Work out the finished part from the listing and answer in its coordinate system (mm). Face numbers are marked on the shaded views. A direction names the side the tool comes from. Give positions to 0.01 mm unless a question says otherwise; leave off trailing zeros. Order: outer loops, then holes, each group sorted by start corner. A loop starts at its lowest first (then second) coordinate and runs counter-clockwise, first axis right, second up. Notation, with made-up numbers: M -26.75,36 L 5.25,36 A18 ccw 5.25,49 Z; hole C 22.5,85 d5. An arc over 180 degrees is marked long. One line per item, written item: value.
from build123d import *

# Parameters (mm, degrees)
F0_W     = 86.995
F0_H     = 86.995
F1_DEPTH = 1.5875
F2_W     = 86.995
F2_H     = 86.995
F2_W_2   = 83.82
F2_H_2   = 83.82
F3_DEPTH = 31.75
F4_R     = 1.7145
F5_DEPTH = 17.78
F6_R     = 2.54
F7_DEPTH = 1.5875


with BuildPart() as f1:
    # F0 (on Top) → F1 (new body)
    with BuildSketch(Plane.XY):
        Rectangle(F0_W, F0_H)
    extrude(amount=F1_DEPTH)

    # F2 (on face) → F3 (join)
    with BuildSketch(Plane.XY.offset(1.5875)):
        Rectangle(F2_W, F2_H)
        Rectangle(F2_W_2, F2_H_2, mode=Mode.SUBTRACT)
    extrude(amount=F3_DEPTH)

    # F4 (on face) → F5 (join)
    with BuildSketch(Plane.XY.offset(1.5875)):
        with BuildLine():
            ThreePointArc((-24.60625, -30.4176050998), (-21.5374457933, -28.6995567884), (-20.32, -25.4))
            ThreePointArc((-20.32, -25.4), (-25.0019007077, -20.3356227477), (-30.4176050998, -24.60625))
            Line((-30.4176050998, -24.60625), (-30.4176050998, -26.19375))
            ThreePointArc((-30.4176050998, -26.19375), (-28.9921024484, -28.9921024484), (-26.19375, -30.4176050998))
            Line((-26.19375, -30.4176050998), (-24.60625, -30.4176050998))
        make_face()
        with Locations((-25.4, -25.4)):
            Circle(F4_R, mode=Mode.SUBTRACT)
        with BuildLine():
            Line((-30.4176050998, -26.19375), (-30.4176050998, -24.60625))
            ThreePointArc((-30.4176050998, -24.60625), (-30.48, -25.4), (-30.4176050998, -26.19375))
        make_face()
        with BuildLine():
            ThreePointArc((-30.4176050998, -26.19375), (-30.48, -25.4), (-30.4176050998, -24.60625))
            Line((-30.4176050998, -24.60625), (-41.91, -24.60625))
            Line((-41.91, -24.60625), (-41.91, -26.19375))
            Line((-41.91, -26.19375), (-30.4176050998, -26.19375))
        make_face()
        with BuildLine():
            Line((-24.60625, -41.91), (-24.60625, -30.4176050998))
            ThreePointArc((-24.60625, -30.4176050998), (-25.4, -30.48), (-26.19375, -30.4176050998))
            Line((-26.19375, -30.4176050998), (-26.19375, -41.91))
            Line((-26.19375, -41.91), (-24.60625, -41.91))
        make_face()
        with BuildLine():
            ThreePointArc((-26.19375, -30.4176050998), (-25.4, -30.48), (-24.60625, -30.4176050998))
            Line((-24.60625, -30.4176050998), (-26.19375, -30.4176050998))
        make_face()
        with BuildLine():
            ThreePointArc((-30.4176050998, 24.60625), (-25.0019007077, 20.3356227477), (-20.32, 25.4))
            ThreePointArc((-20.32, 25.4), (-21.5374457933, 28.6995567884), (-24.60625, 30.4176050998))
            ThreePointArc((-24.60625, 30.4176050998), (-25.4, 30.48), (-26.19375, 30.4176050998))
            ThreePointArc((-26.19375, 30.4176050998), (-28.9921024484, 28.9921024484), (-30.4176050998, 26.19375))
            ThreePointArc((-30.4176050998, 26.19375), (-30.48, 25.4), (-30.4176050998, 24.60625))
        make_face()
        with Locations((-25.4, 25.4)):
            Circle(F4_R, mode=Mode.SUBTRACT)
        with BuildLine():
            ThreePointArc((-26.19375, 30.4176050998), (-25.4, 30.48), (-24.60625, 30.4176050998))
            Line((-24.60625, 30.4176050998), (-24.60625, 41.91))
            Line((-24.60625, 41.91), (-26.19375, 41.91))
            Line((-26.19375, 41.91), (-26.19375, 30.4176050998))
        make_face()
        with BuildLine():
            Line((-41.91, 24.60625), (-30.4176050998, 24.60625))
            ThreePointArc((-30.4176050998, 24.60625), (-30.48, 25.4), (-30.4176050998, 26.19375))
            Line((-30.4176050998, 26.19375), (-41.91, 26.19375))
            Line((-41.91, 26.19375), (-41.91, 24.60625))
        make_face()
        with BuildLine():
            Line((24.60625, -41.91), (26.19375, -41.91))
            Line((26.19375, -41.91), (26.19375, -30.4176050998))
            ThreePointArc((26.19375, -30.4176050998), (25.4, -30.48), (24.60625, -30.4176050998))
            Line((24.60625, -30.4176050998), (24.60625, -41.91))
        make_face()
        with BuildLine():
            ThreePointArc((24.60625, -30.4176050998), (25.4, -30.48), (26.19375, -30.4176050998))
            ThreePointArc((26.19375, -30.4176050998), (28.9921024484, -28.9921024484), (30.4176050998, -26.19375))
            ThreePointArc((30.4176050998, -26.19375), (30.4643772523, -25.7980992923), (30.48, -25.4))
            ThreePointArc((30.48, -25.4), (30.4643772523, -25.0019007077), (30.4176050998, -24.60625))
            ThreePointArc((30.4176050998, -24.60625), (21.8078975516, -21.8078975516), (24.60625, -30.4176050998))
        make_face()
        with Locations((25.4, -25.4)):
            Circle(F4_R, mode=Mode.SUBTRACT)
        with BuildLine():
            ThreePointArc((30.48, -25.4), (30.4643772523, -25.7980992923), (30.4176050998, -26.19375))
            Line((30.4176050998, -26.19375), (41.91, -26.19375))
            Line((41.91, -26.19375), (41.91, -24.60625))
            Line((41.91, -24.60625), (30.4176050998, -24.60625))
            ThreePointArc((30.4176050998, -24.60625), (30.4643772523, -25.0019007077), (30.48, -25.4))
        make_face()
        with BuildLine():
            Line((30.4176050998, 24.60625), (41.91, 24.60625))
            Line((41.91, 24.60625), (41.91, 26.19375))
            Line((41.91, 26.19375), (30.4176050998, 26.19375))
            ThreePointArc((30.4176050998, 26.19375), (30.4643772523, 25.7980992923), (30.48, 25.4))
            ThreePointArc((30.48, 25.4), (30.4643772523, 25.0019007077), (30.4176050998, 24.60625))
        make_face()
        with BuildLine():
            ThreePointArc((24.60625, 30.4176050998), (21.8078975516, 21.8078975516), (30.4176050998, 24.60625))
            ThreePointArc((30.4176050998, 24.60625), (30.4643772523, 25.0019007077), (30.48, 25.4))
            ThreePointArc((30.48, 25.4), (30.4643772523, 25.7980992923), (30.4176050998, 26.19375))
            ThreePointArc((30.4176050998, 26.19375), (28.9921024484, 28.9921024484), (26.19375, 30.4176050998))
            ThreePointArc((26.19375, 30.4176050998), (25.4, 30.48), (24.60625, 30.4176050998))
        make_face()
        with Locations((25.4, 25.4)):
            Circle(F4_R, mode=Mode.SUBTRACT)
        with BuildLine():
            Line((24.60625, 41.91), (24.60625, 30.4176050998))
            ThreePointArc((24.60625, 30.4176050998), (25.4, 30.48), (26.19375, 30.4176050998))
            Line((26.19375, 30.4176050998), (26.19375, 41.91))
            Line((26.19375, 41.91), (24.60625, 41.91))
        make_face()
    extrude(amount=F5_DEPTH)

    # F6 (on face) → F7 (cut, through all)
    with BuildSketch(Plane.YZ.offset(43.4975)):
        with Locations((0, 25.4)):
            Circle(F6_R)
        with Locations((0, 6.35)):
            Circle(F6_R)
    extrude(amount=-F7_DEPTH, mode=Mode.SUBTRACT)


solid = f1.part
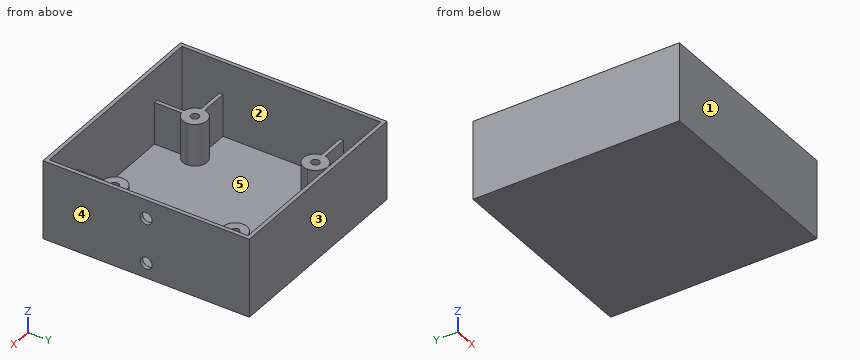
(1) Given P1, Ø5.5, axis at x = -25.4, y = -25.4, coming from the +Z side; P2, Ø4, axis at x = 27.5, y = 18.5, coming from the +Z side, each flat-ended and moving along its own axis, determine where each tip first touches the part or whether it passes through.
Findings:
P1: stops at z = 19.37
P2: stops at z = 1.59
(2) Find the intervals of material crossed by probe 1 along X at (y, z) = (-32, 14); probe 2 along Y at (x, z) = (25.4, 9.5), in increasing order. Write a range as from..to.
Findings:
probe 1: x = -43.5..-41.91, -26.19..-24.61, 24.61..26.19, 41.91..43.5
probe 2: y = -43.5..-27.11, -23.69..-20.32, 20.32..23.69, 27.11..43.5
(3) Section C-C, the plane z = 25.4 is taken. Give the vertices of the cut face in (x, y), then the cut area to 3 significant figures.
Findings:
outline: M -43.5,-43.5 L 43.5,-43.5 L 43.5,-2.54 L 41.91,-2.54 L 41.91,-41.91 L -41.91,-41.91 L -41.91,41.91 L 41.91,41.91 L 41.91,2.54 L 43.5,2.54 L 43.5,43.5 L -43.5,43.5 Z
area: 534 mm^2
(4) Determine the mould class of the marked faces 3, 4 and 5 for opening direction X: pulls with the +X half, pulls with the -X half, needs draft (parallel to the pull), parting line crosses it, or undercut.
Findings:
face 3: needs draft
face 4: pulls with the +X half
face 5: undercut
(5) Section A-A, the plane y = 0 is taken. Give the vertices of the cut face in (x, z), then the cut area to 3 significant figures.
Findings:
outline: M -43.5,0 L 43.5,0 L 43.5,3.81 L 41.91,3.81 L 41.91,1.59 L -41.91,1.59 L -41.91,33.34 L -43.5,33.34 Z; M 41.91,8.89 L 43.5,8.89 L 43.5,22.86 L 41.91,22.86 Z; M 41.91,27.94 L 43.5,27.94 L 43.5,33.34 L 41.91,33.34 Z
area: 223 mm^2
(6) Which of the six approach directions +Z, -Z, +X, -X, +Y, -Y give full straight-line access (tool end or side, diameter ignored) to the marked faces 1 and 2?
Findings:
face 1: +Z, -Z, +X, -X, -Y
face 2: +Z
(7) Section B-B, the plane x = 36 is taken. Give the vertices of the cut face in (y, z).
Findings:
outline: M -43.5,0 L 43.5,0 L 43.5,33.34 L 41.91,33.34 L 41.91,1.59 L 26.19,1.59 L 26.19,19.37 L 24.61,19.37 L 24.61,1.59 L -24.61,1.59 L -24.61,19.37 L -26.19,19.37 L -26.19,1.59 L -41.91,1.59 L -41.91,33.34 L -43.5,33.34 Z
(8) Section D-D, the plane y = 22.5 is taken. Give the vertices of the cut face in (x, z).
Findings:
outline: M -43.5,0 L 43.5,0 L 43.5,33.34 L 41.91,33.34 L 41.91,1.59 L 29.57,1.59 L 29.57,19.37 L 21.23,19.37 L 21.23,1.59 L -21.23,1.59 L -21.23,19.37 L -29.57,19.37 L -29.57,1.59 L -41.91,1.59 L -41.91,33.34 L -43.5,33.34 Z
